The listing builds one solid part. Answer for the finished solid, in the listing's coordinates (mm). A direction names the side the tool comes from. Coordinates: 2 decimals unless noted, no trailing zeros. One line per question, with ' | ' between items.
from build123d import *

# Parameters (mm, degrees)
SKETCH1_W            = 180
SKETCH1_H            = 160
BOSS_EXTRUDE1_DEPTH  = 3
BOSS_EXTRUDE2_DEPTH  = 10
FILLET1_START        = -47
FILLET1_DEPTH        = 94
FILLET1_2_DEPTH      = 4
FILLET1_START_2      = 43
FILLET1_3_DEPTH      = 4
M3_CLEARANCE_HOLE1_D = 3.4


with BuildPart() as part:
    # Sketch1 → Boss-Extrude1 (new body)
    with BuildSketch(Plane(origin=(0, 0, 0), x_dir=(1, 0, 0), z_dir=(0, 1, 0))):
        Rectangle(SKETCH1_W, SKETCH1_H)
        with BuildLine():
            Line((-80, -58.195), (-76, -58.195))
            ThreePointArc((-76, -58.195), (-74.445, -59.75), (-76, -61.305))
            Line((-76, -61.305), (-80, -61.305))
            ThreePointArc((-80, -61.305), (-81.555, -59.75), (-80, -58.195))
        make_face(mode=Mode.SUBTRACT)
        with BuildLine():
            Line((-58, -58.195), (-54, -58.195))
            ThreePointArc((-54, -58.195), (-52.445, -59.75), (-54, -61.305))
            Line((-54, -61.305), (-58, -61.305))
            ThreePointArc((-58, -61.305), (-59.555, -59.75), (-58, -58.195))
        make_face(mode=Mode.SUBTRACT)
        with BuildLine():
            Line((-80, -71.695), (-76, -71.695))
            ThreePointArc((-76, -71.695), (-74.445, -73.25), (-76, -74.805))
            Line((-76, -74.805), (-80, -74.805))
            ThreePointArc((-80, -74.805), (-81.555, -73.25), (-80, -71.695))
        make_face(mode=Mode.SUBTRACT)
        with BuildLine():
            Line((-58, -71.695), (-54, -71.695))
            ThreePointArc((-54, -71.695), (-52.445, -73.25), (-54, -74.805))
            Line((-54, -74.805), (-58, -74.805))
            ThreePointArc((-58, -74.805), (-59.555, -73.25), (-58, -71.695))
        make_face(mode=Mode.SUBTRACT)
        with BuildLine():
            Line((-80, 71.695), (-76, 71.695))
            ThreePointArc((-76, 71.695), (-74.445, 73.25), (-76, 74.805))
            Line((-76, 74.805), (-80, 74.805))
            ThreePointArc((-80, 74.805), (-81.555, 73.25), (-80, 71.695))
        make_face(mode=Mode.SUBTRACT)
        with BuildLine():
            Line((-58, 71.695), (-54, 71.695))
            ThreePointArc((-54, 71.695), (-52.445, 73.25), (-54, 74.805))
            Line((-54, 74.805), (-58, 74.805))
            ThreePointArc((-58, 74.805), (-59.555, 73.25), (-58, 71.695))
        make_face(mode=Mode.SUBTRACT)
        with BuildLine():
            Line((-58, 58.195), (-54, 58.195))
            ThreePointArc((-54, 58.195), (-52.445, 59.75), (-54, 61.305))
            Line((-54, 61.305), (-58, 61.305))
            ThreePointArc((-58, 61.305), (-59.555, 59.75), (-58, 58.195))
        make_face(mode=Mode.SUBTRACT)
        with BuildLine():
            Line((-80, 58.195), (-76, 58.195))
            ThreePointArc((-76, 58.195), (-74.445, 59.75), (-76, 61.305))
            Line((-76, 61.305), (-80, 61.305))
            ThreePointArc((-80, 61.305), (-81.555, 59.75), (-80, 58.195))
        make_face(mode=Mode.SUBTRACT)
        with BuildLine():
            Line((80, -71.695), (76, -71.695))
            ThreePointArc((76, -71.695), (74.445, -73.25), (76, -74.805))
            Line((76, -74.805), (80, -74.805))
            ThreePointArc((80, -74.805), (81.555, -73.25), (80, -71.695))
        make_face(mode=Mode.SUBTRACT)
        with BuildLine():
            Line((80, -58.195), (76, -58.195))
            ThreePointArc((76, -58.195), (74.445, -59.75), (76, -61.305))
            Line((76, -61.305), (80, -61.305))
            ThreePointArc((80, -61.305), (81.555, -59.75), (80, -58.195))
        make_face(mode=Mode.SUBTRACT)
        with BuildLine():
            Line((58, -58.195), (54, -58.195))
            ThreePointArc((54, -58.195), (52.445, -59.75), (54, -61.305))
            Line((54, -61.305), (58, -61.305))
            ThreePointArc((58, -61.305), (59.555, -59.75), (58, -58.195))
        make_face(mode=Mode.SUBTRACT)
        with BuildLine():
            Line((58, -71.695), (54, -71.695))
            ThreePointArc((54, -71.695), (52.445, -73.25), (54, -74.805))
            Line((54, -74.805), (58, -74.805))
            ThreePointArc((58, -74.805), (59.555, -73.25), (58, -71.695))
        make_face(mode=Mode.SUBTRACT)
        with BuildLine():
            Line((80, 58.195), (76, 58.195))
            ThreePointArc((76, 58.195), (74.445, 59.75), (76, 61.305))
            Line((76, 61.305), (80, 61.305))
            ThreePointArc((80, 61.305), (81.555, 59.75), (80, 58.195))
        make_face(mode=Mode.SUBTRACT)
        with BuildLine():
            Line((58, 58.195), (54, 58.195))
            ThreePointArc((54, 58.195), (52.445, 59.75), (54, 61.305))
            Line((54, 61.305), (58, 61.305))
            ThreePointArc((58, 61.305), (59.555, 59.75), (58, 58.195))
        make_face(mode=Mode.SUBTRACT)
        with BuildLine():
            Line((58, 71.695), (54, 71.695))
            ThreePointArc((54, 71.695), (52.445, 73.25), (54, 74.805))
            Line((54, 74.805), (58, 74.805))
            ThreePointArc((58, 74.805), (59.555, 73.25), (58, 71.695))
        make_face(mode=Mode.SUBTRACT)
        with BuildLine():
            Line((80, 71.695), (76, 71.695))
            ThreePointArc((76, 71.695), (74.445, 73.25), (76, 74.805))
            Line((76, 74.805), (80, 74.805))
            ThreePointArc((80, 74.805), (81.555, 73.25), (80, 71.695))
        make_face(mode=Mode.SUBTRACT)
    extrude(amount=BOSS_EXTRUDE1_DEPTH)

    # Sketch1<3> → Boss-Extrude2 (add)
    with BuildSketch(Plane(origin=(0, 0, 0), x_dir=(1, 0, 0), z_dir=(0, 1, 0))):
        Polygon((-70, 47), (-70, 43), (70, 43), (70, -43), (-70, -43), (-70, -47), (74, -47), (74, 47), align=None)
    extrude(amount=BOSS_EXTRUDE2_DEPTH)

    # Fillet1: read off the stored shape, not the designer's step
    # Fillet1 outline → Fillet1 (add)
    with BuildSketch(Plane.XY.offset(FILLET1_START)):
        with BuildLine():
            Line((74, 10), (74, 3))
            Line((74, 3), (83.539392014, 3))
            add(Edge.make_bspline(
                [(83.539392014, 3), (82.252081476, 3), (80.964770938, 3), (78.099649509, 3.423086243), (76.035521304, 4.937742252), (74.772386323, 7.543968027), (74.386193161, 8.771984013), (74, 10)],
                knots=[0, 0, 0, 0, 0, 0, 0.5, 0.5, 1, 1, 1, 1, 1, 1], degree=5))
        make_face()
    extrude(amount=FILLET1_DEPTH)

    # Fillet1 2 outline → Fillet1 2 (add)
    with BuildSketch(Plane.XY.offset(FILLET1_START)):
        with BuildLine():
            add(Edge.make_bspline(
                [(-79.539392014, 3), (-78.252081476, 3), (-76.964770938, 3), (-74.099649509, 3.423086243), (-72.035521304, 4.937742252), (-70.772386323, 7.543968027), (-70.386193161, 8.771984013), (-70, 10)],
                knots=[0, 0, 0, 0, 0, 0, 0.5, 0.5, 1, 1, 1, 1, 1, 1], degree=5))
            Line((-79.539392014, 3), (-70, 3))
            Line((-70, 3), (-70, 10))
        make_face()
    extrude(amount=FILLET1_2_DEPTH)

    # Fillet1 3 outline → Fillet1 3 (add)
    with BuildSketch(Plane.XY.offset(FILLET1_START_2)):
        with BuildLine():
            add(Edge.make_bspline(
                [(-79.539392014, 3), (-78.252081476, 3), (-76.964770938, 3), (-74.099649509, 3.423086243), (-72.035521304, 4.937742252), (-70.772386323, 7.543968027), (-70.386193161, 8.771984013), (-70, 10)],
                knots=[0, 0, 0, 0, 0, 0, 0.5, 0.5, 1, 1, 1, 1, 1, 1], degree=5))
            Line((-79.539392014, 3), (-70, 3))
            Line((-70, 3), (-70, 10))
        make_face()
    extrude(amount=FILLET1_3_DEPTH)

    # M3 Clearance Hole1 (through all)
    with Locations(Plane(origin=(0, 3, 0), x_dir=(1, 0, 0), z_dir=(0, 1, 0))):
        with Locations((-44, -66.5), (-34, -66.5), (-24, -66.5), (-14, -66.5), (-4, -66.5), (6, -66.5), (16, -66.5), (26, -66.5), (36, -66.5), (46, -66.5), (46, 66.5), (36, 66.5), (26, 66.5), (16, 66.5), (6, 66.5), (-4, 66.5), (-14, 66.5), (-24, 66.5), (-34, 66.5), (-44.881291433, 66.5)):
            Hole(M3_CLEARANCE_HOLE1_D / 2)


solid = part.part
Item 1: Find the intervals of material crossed by line 1 (Z direction, x = -24, y = 0.6); line 2 (Z direction, x = 54.5, y = 2) (3 decimals); line 3 (Z direction, x = -37, y = 8), in increasing order. Write a range as [from, to].
Taken from the geometry:
line 1: z = [-80, -68.2], [-64.8, 64.8], [68.2, 80] | line 2: z = [-80, -74.805], [-71.695, -61.305], [-58.195, 58.195], [61.305, 71.695], [74.805, 80] | line 3: z = [-47, -43], [43, 47]
Item 2: Each of these flat-tipped pins is pushed along its axis until it touches: pin 1 Ø6 at (y, z) = (8.5, 48) entering from -X; pin 2 Ø2.5 at (x, z) = (-24, -66.5) entering from -Y; pin 3 Ø2 at (x, z) = (67.5, 15.5) entering from +Y; pin 4 Ø8 at (x, z) = (63, -28.5) entering from -Y. Where does it stop, or does it pass through?
Taken from the geometry:
pin 1: stops at x = -72.02 | pin 2: passes through | pin 3: stops at y = 3 | pin 4: stops at y = 0
Item 3: The mould has two halves that part along Z. Classify faces 1 (the face through (-4, 7, 43)), 2 (the face through (3, 7, -47)), 3 (the face through (-1, 0, -1)): pulls with the +Z half, pulls with the -Z half, needs draft (parallel to the pull), parting line crosses it, or undercut.
Taken from the geometry:
face 1: undercut | face 2: pulls with the -Z half | face 3: needs draft
Item 4: Which of the six approach directions +Z, -Z, +X, -X, +Y, -Y give full straight-line access (tool end or side, diameter ignored) to faces 4 (the face through (-4, 7, -43)), 5 (the face through (3, 7, 47)), 6 (the face through (23, 10, 45))?
Taken from the geometry:
face 4: -X, +Y | face 5: +Z, +X, -X, +Y | face 6: +Z, -Z, +X, -X, +Y
